Check sheet for the modelled part. Datum: model origin and axes. Units: mm. Face numbers are marked on the shaded views. Give positions to 0.01 mm unless a question says otherwise; leave off trailing zeros. Loops run counter-clockwise (first coordinate to the right, second up) from the corner with the lowest first, then second, coordinate; pieces in that order, holes last. Notation, with made-up numbers: (9.5, -22) - (63.5, -22) arc R19 cw to (63.5, 11) - close; hole circle Ø2 at (-17, 78.5). An arc over 180 degrees is marked (long way). Answer in a Markdown table with one row per item. Add a question column.
(1) Thickness scan on L1, parallel to Z at x = 0, y = -4.25; L2, parallel to X at y = -7, z = 3; L3, parallel to Z at x = -7, y = -9.25. Record the ranges inside material, lowest first.
(2) Sectioned sample at A-A on y = -3.5. Enter the section's corners in (x, z).
(3) Go/stop test with a flat-tipped pin: P1, Ø5, axis at y = -8.5, z = -18.5, coming from the +X side. Record where the tip stops, or that it passes through.
(4) Draft check along X on the marked faces 1, 2 and 3. Enter one of: released by +X, released by -X, zero draft, split by the parting line, or undercut.
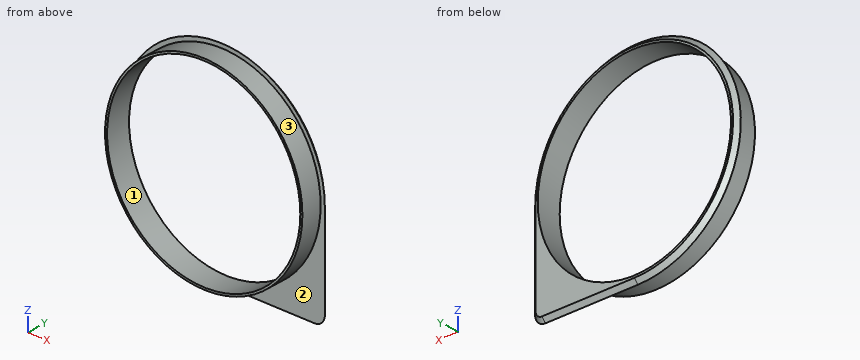
from build123d import *

# Parameters (mm, degrees)
F0_R     = 47.5
F0_R_2   = 46.5
F1_DEPTH = 2
F2_DEPTH = 12
F3_SIZE  = 1.99999


# Not quite as in the source:
# - a fillet or chamfer is up to 0.001 mm smaller than in the source, because OpenCascade refuses the exact size


with BuildPart() as f1:
    # F0 (on Front) → F1 (new body)
    with BuildSketch(Plane.XZ):
        with BuildLine():
            ThreePointArc((0, -49.5), (35.0017856687, -35.0017856687), (49.5, 0))
            ThreePointArc((49.5, 0), (-35.0017856687, 35.0017856687), (0, -49.5))
        make_face()
        Circle(F0_R, mode=Mode.SUBTRACT)
        Circle(F0_R)
        Circle(F0_R_2, mode=Mode.SUBTRACT)
        with BuildLine():
            Line((49.5, -44.5), (49.5, 0))
            ThreePointArc((49.5, 0), (35.0017856687, -35.0017856687), (0, -49.5))
            Line((0, -49.5), (44.5, -49.5))
            ThreePointArc((44.5, -49.5), (48.0355339059, -48.0355339059), (49.5, -44.5))
        make_face()
    extrude(amount=F1_DEPTH)

    # F0 (on Front) → F2 (join)
    with BuildSketch(Plane.XZ):
        Circle(F0_R)
        Circle(F0_R_2, mode=Mode.SUBTRACT)
    extrude(amount=F2_DEPTH)

    # F3 (size 2 in the source; OpenCascade refuses exactly that, so slightly less here)
    f3_edges = [f1.edges().sort_by_distance(p)[0] for p in [
        (49.5, 0, -22.25),
    ]]
    chamfer(f3_edges, length=F3_SIZE)


solid = f1.part
Reply:
| question | item | result |
|---|---|---|
| 1 | L1 | -47.5 to -46.5, 46.5 to 47.5 |
| 1 | L2 | -47.41 to -46.4, 46.4 to 47.41 |
| 1 | L3 | -46.98 to -45.97, 45.97 to 46.98 |
| 2 | outline | circle Ø95 at (0, 0); hole circle Ø93 at (0, 0) |
| 3 | P1 | x = 44.72 |
| 4 | face 1 | undercut |
| 4 | face 2 | zero draft |
| 4 | face 3 | split by the parting line |
